Input: part model. Units: mm. Frame: model coordinates. Round coordinates to 2 decimals unless told otherwise and drop trailing zeros. Loops run counter-clockwise (first coordinate to the right, second up) from the corner with the lowest first, then second, coordinate; pieces in that order, holes last. Notation, with made-up numbers: (84, 7.25) -> (128, 7.25) arc R23 cw to (128, 45.25) -> close; hole circle Ø2 at (66.25, 65.25). An arc over 180 degrees is marked (long way). Answer as a JSON object with one key per item and string values.
```python
from build123d import *

# Parameters (mm, degrees)
SKETCH_1_W          = 60
SKETCH_1_H          = 60
SKETCH_1_R          = 1.5
EXTRUDE_1_DEPTH     = 3
SKETCH_2_R          = 1.5
CUT_EXTRUDE_1_DEPTH = 10
FILLET_1_R          = 2


with BuildPart() as part:
    # 草图1 → 凸台-拉伸1 (new body)
    with BuildSketch(Plane(origin=(0, 0, 0), x_dir=(1, 0, 0), z_dir=(0, 1, 0))):
        Rectangle(SKETCH_1_W, SKETCH_1_H)
        with Locations(Location((-5, 27, 0), (0, 0, 270))):
            Circle(SKETCH_1_R, mode=Mode.SUBTRACT)
        with Locations(Location((15, 27, 0), (0, 0, 270))):
            Circle(SKETCH_1_R, mode=Mode.SUBTRACT)
        with Locations(Location((15, -27, 0), (0, 0, 90))):
            Circle(SKETCH_1_R, mode=Mode.SUBTRACT)
        with Locations(Location((-5, -27, 0), (0, 0, 90))):
            Circle(SKETCH_1_R, mode=Mode.SUBTRACT)
        with Locations(Location((-25, 0, 0), (0, 0, 270))):
            Circle(SKETCH_1_R, mode=Mode.SUBTRACT)
        with Locations(Location((25, 0, 0), (0, 0, 270))):
            Circle(SKETCH_1_R, mode=Mode.SUBTRACT)
    extrude(amount=EXTRUDE_1_DEPTH)

    # 草图2 → 切除-拉伸1 (cut)
    with BuildSketch(Plane(origin=(0, 3, 0), x_dir=(1, 0, 0), z_dir=(0, 1, 0))):
        with Locations(Location((-25, 25, 0), (0, 0, 270))):
            Circle(SKETCH_2_R)
        with Locations(Location((25, 25, 0), (0, 0, 270))):
            Circle(SKETCH_2_R)
        with Locations(Location((-25, -25, 0), (0, 0, 270))):
            Circle(SKETCH_2_R)
        with Locations(Location((25, -25, 0), (0, 0, 270))):
            Circle(SKETCH_2_R)
    extrude(amount=-CUT_EXTRUDE_1_DEPTH, mode=Mode.SUBTRACT)

    # 圆角1
    fillet_1_edges = [part.edges().sort_by_distance(p)[0] for p in [
        (30, 1.5, 30),
        (-30, 1.5, 30),
        (-30, 1.5, -30),
        (30, 1.5, -30),
    ]]
    fillet(fillet_1_edges, radius=FILLET_1_R)


solid = part.part
```
1) Ray query, probe 1 along X at (y, z) = (1.5, -25); probe 2 along X at (y, z) = (1.6, -27). Return the intervals inside material, ascending.
Output:
{"probe 1": "x = -30 to -26.5, -23.5 to 23.5, 26.5 to 30", "probe 2": "x = -30 to -6.5, -3.5 to 13.5, 16.5 to 30"}
2) Section B-B, the plane x = 15. Output: boundary loops of the cut face in (y, z), plus the area to 3 significant figures.
Output:
{"outline": "(0, -30) -> (3, -30) -> (3, -28.5) -> (0, -28.5) -> close; (0, -25.5) -> (3, -25.5) -> (3, 25.5) -> (0, 25.5) -> close; (0, 28.5) -> (3, 28.5) -> (3, 30) -> (0, 30) -> close", "area": "162 mm^2"}
3) Draft query along Z for faces 1 (the face through (0, 1, -30)), 2 (the face through (-29.43, 1.52, 29.4)), 3 (the face through (26.487, 1.479, -0.195)). Return one class per face: +Z half, -Z half, draft (parallel to the pull), parting line (faces both ways), or undercut.
Output:
{"face 1": "-Z half", "face 2": "+Z half", "face 3": "undercut"}
4) Section D-D, the plane x = -25. Output: boundary loops of the cut face in (y, z).
Output:
{"outline": "(0, -30) -> (3, -30) -> (3, -26.5) -> (0, -26.5) -> close; (0, -23.5) -> (3, -23.5) -> (3, -1.5) -> (0, -1.5) -> close; (0, 1.5) -> (3, 1.5) -> (3, 23.5) -> (0, 23.5) -> close; (0, 26.5) -> (3, 26.5) -> (3, 30) -> (0, 30) -> close"}
5) Section A-A, the plane z = 0. Output: boundary loops of the cut face in (x, y), plus the area to 3 significant figures.
Output:
{"outline": "(-30, 0) -> (-26.5, 0) -> (-26.5, 3) -> (-30, 3) -> close; (-23.5, 0) -> (23.5, 0) -> (23.5, 3) -> (-23.5, 3) -> close; (26.5, 0) -> (30, 0) -> (30, 3) -> (26.5, 3) -> close", "area": "162 mm^2"}
6) Section C-C, the plane y = 1.3. Count the separate pieces of the cut face and the enclosed holes in it, plus the area to 3 significant figures.
Output:
{"separate pieces": "1", "enclosed holes": "10", "area": "3,530 mm^2"}
